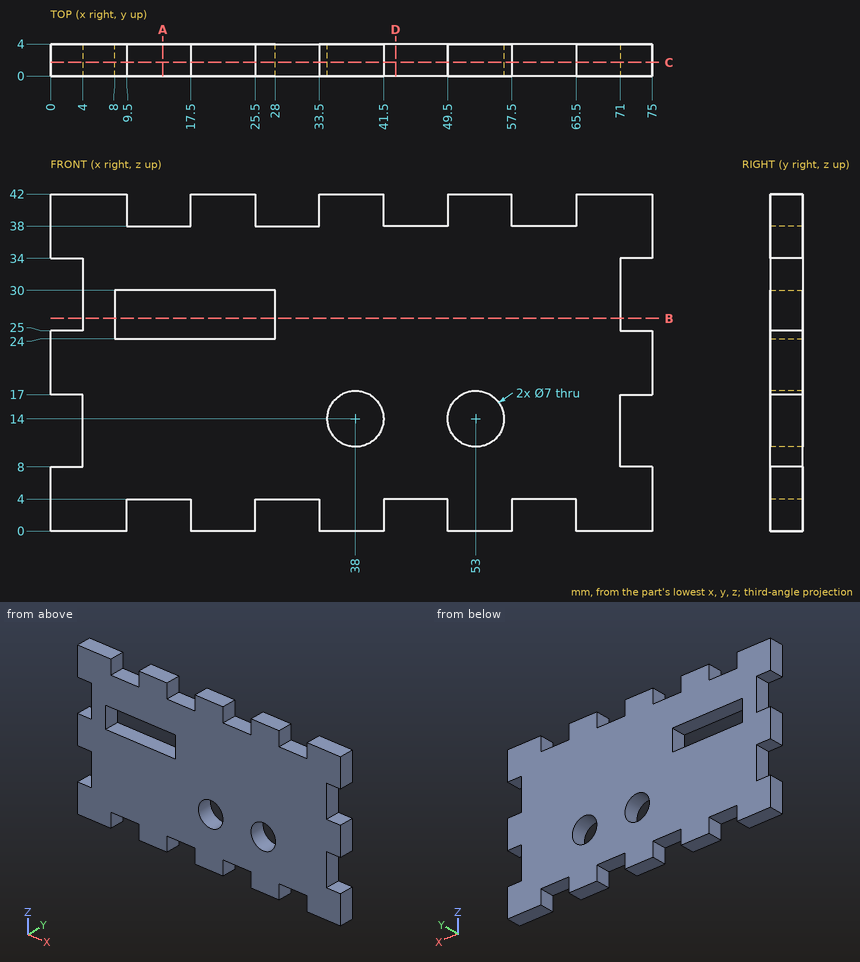
Input: dimensioned drawing with shaded views. Units: mm. Origin: part minimum x, y, z. Coordinates: 2 decimals unless noted, no trailing zeros. Order: outer loops, then holes, each group sorted by start corner. A loop starts at its lowest first (then second) coordinate and runs counter-clockwise, first axis right, second up.
(1) Section query A-A (x = 14). Return the cut outline in (y, z).
(2) Section query B-B (z = 26.5). Return the cut outline in (x, y).
(3) First-contact query: pin 1 (4 mm diameter, centred on x = 29, z = 10, fed in from -Y); pin 2 (1.2 mm diameter, centred on x = 13, y = 2, fed in from -Z); pin 3 (2 mm diameter, centred on y = 1, z = 27.5, fed in from +X); pin 4 (1.2 mm diameter, centred on y = 1.5, z = 26, fed in from -X). Flat tips, straight axial feed; report the tip coordinate or a pass-through.
(4) Section query C-C (y = 1.7). State how many separate pieces and enclosed holes the cut face has, plus the area to 3 significant figures.
(5) Material intervals for probe 1 along X at (y, z) = (1.5, 13); probe 2 along Z at (x, y) = (17, 3.7); probe 3 along Z at (x, y) = (38, 2.85), sorted ascending.
(6) Section query D-D (x = 43). Return the cut outline in (y, z).
Solution:
1. outline: (0, 4) - (4, 4) - (4, 24) - (0, 24) - close; (0, 30) - (4, 30) - (4, 38) - (0, 38) - close
2. outline: (4, 0) - (8, 0) - (8, 4) - (4, 4) - close; (28, 0) - (71, 0) - (71, 4) - (28, 4) - close
3. pin 1: stops at y = 0
3. pin 2: stops at z = 4
3. pin 3: stops at x = 71
3. pin 4: stops at x = 4
4. separate pieces: 1
4. enclosed holes: 3
4. area: 2,550 mm2
5. probe 1: x = 4 to 34.65, 41.35 to 49.65, 56.35 to 71
5. probe 2: z = 4 to 24, 30 to 38
5. probe 3: z = 0 to 10.5, 17.5 to 42
6. outline: (0, 4) - (4, 4) - (4, 38) - (0, 38) - close
